Verification items for the finished model (mm, model axes). A direction names the side the tool comes from. Give positions to 0.01 mm unless a question says otherwise; leave off trailing zeros. Write each loop counter-clockwise with the first axis right and the second up, starting at its lowest first coordinate (ties: lowest second). Pieces come first, ordered by that corner, then holes. Notation, with made-up numbers: (82, 71) - (95, 71) arc R19 cw to (95, 78) - close; hole circle Ø1 at (80, 37.5). An arc over 180 degrees is marked (long way). Answer as a JSON object with one key per item and string values. Group by question number.
Item 1: Go/stop test with flat-tipped pins: pin 1 (6 mm diameter, centred on x = 4, y = 36.5, fed in from -Z); pin 2 (10 mm diameter, centred on y = 48, z = -7, fed in from -X); pin 3 (1.5 mm diameter, centred on x = -3, y = 27.5, fed in from +Z). Record where each tip stops, or that it passes through.
Item 2: Tool access check on faces 5 (the face through (4, 4, -11)), 6 (the face through (-2, 76, 2)), 7 (the face through (0, 80, 0)). Record the directions out of +Z, -Z, +X, -X, +Y, -Y that give a thin tool (end or side, any length) a straight path to the whole face; none if there is none.
Item 3: Sectioned sample at C-C, the plane y = 19.5. Record the boundary of the cut face in (x, z), and give its area (3 significant figures).
Item 4: Draft check along Y on faces 1 (the face through (-0.54, 74.99, -2.44)), 2 (the face through (-3.72, 3.84, -16.75)), 3 (the face through (0, 0, 0)), 4 (the face through (-2.539, 0.76, -19.334)). Enter one of: +Y half, -Y half, draft (parallel to the pull), parting line (faces both ways), or undercut.
Item 5: Sectioned sample at B-B, the plane z = 0. Record the boundary of the cut face in (x, y).
Item 6: Scan lines: line 1 along Y through (x, z) = (-9.5, 5); line 2 along Y through (x, z) = (2, 3.5); line 3 along Z through (x, y) = (-2.5, 34). Record each from-to range of solid material in increasing order. Write a range as [from, to].
Item 7: Sectioned sample at A-A, the plane x = 0. Record the boundary of the cut face in (y, z).
Autodesk Inventor part; units mm, degrees
ref_plane "YZ Plane" through (0, 0, 0) normal (1, 0, 0) x (0, 1, 0)
ref_plane "XZ Plane" through (0, 0, 0) normal (0, 1, 0) x (-1, 0, 0)
ref_plane "XY Plane" through (0, 0, 0) normal (0, 0, 1) x (1, 0, 0)
sketch "Эскиз1" plane through (0, 0, 0) normal (0, 0, 1) x (1, 0, 0)
  line L0 (0, 0) -> (19.5, 0)
  line L1 (19.5, 0) -> (19.5, 1.5)
  line L2 (19.5, 1.5) -> (17, 4)
  line L3 (0, 80) -> (3, 80)
  line L4 (17, 4) -> (11, 4)
  arc A0 (3, 12) -> (11, 4) centre (11, 12) ccw
  line L5 (3, 80) -> (3, 76)
  line L6 (3, 76) -> (2.5, 76)
  line L7 (2.5, 76) -> (2.5, 74)
  line L8 (2.5, 74) -> (3, 74)
  line L9 (3, 80) -> (3, 76)
  line L10 (3, 74) -> (3, 12)
  line L11 (0, 80) -> (0, 0)
  dimension "d0" = 19.5
  dimension "d1" = 1.5
  dimension "d2" = 45
  dimension "d3" = 17
  dimension "d4" = 3
  dimension "d5" = 8
  dimension "d6" = 80
  dimension "d7" = 4
  dimension "d8" = 2
  dimension "d9" = 0.5
revolve "Вращение1" add sketch "Эскиз1" angle 360 about axis through (0, 80, 0) along (0, -1, 0)
properties part number "выпускной_клапан"
Geometry check:
{
 "1": {"pin 1": "z = -2.83", "pin 2": "x = -2.24", "pin 3": "z = 1.98"},
 "2": {"face 5": "+Y", "face 6": "none", "face 7": "+Z, -Z, +X, -X, +Y"},
 "3": {"outline": "circle Ø6 at (0, 0)", "area": "28.3 mm^2"},
 "4": {"face 1": "undercut", "face 2": "+Y half", "face 3": "-Y half", "face 4": "draft"},
 "5": {"outline": "(-19.5, 0) - (19.5, 0) - (19.5, 1.5) - (17, 4) - (11, 4) arc R8 cw to (3, 12) - (3, 74) - (2.5, 74) - (2.5, 76) - (3, 76) - (3, 80) - (-3, 80) - (-3, 76) - (-2.5, 76) - (-2.5, 74) - (-3, 74) - (-3, 12) arc R8 cw to (-11, 4) - (-17, 4) - (-19.5, 1.5) - close"},
 "6": {"line 1": "[0, 4]", "line 2": "[0, 8.07]", "line 3": "[-1.66, 1.66]"},
 "7": {"outline": "(0, -19.5) - (1.5, -19.5) - (4, -17) - (4, -11) arc R8 cw to (12, -3) - (74, -3) - (74, -2.5) - (76, -2.5) - (76, -3) - (80, -3) - (80, 3) - (76, 3) - (76, 2.5) - (74, 2.5) - (74, 3) - (12, 3) arc R8 cw to (4, 11) - (4, 17) - (1.5, 19.5) - (0, 19.5) - close"}
}
